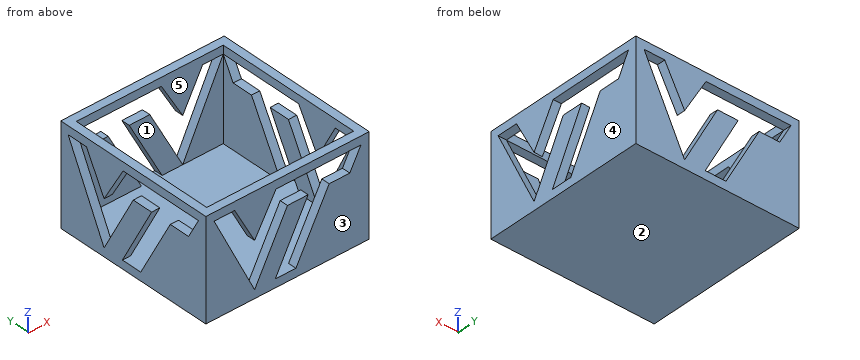
from build123d import *

# Parameters (mm, degrees)
F1_W      = 50.238024
F1_H      = 30.48
F2_DEPTH  = 50.2412
F4_T      = -2.54
F7_DEPTH  = 2.54
F8_DEPTH  = 2.54
F9_DEPTH  = 2.54
F10_DEPTH = 2.54


with BuildPart() as f2:
    # F1 (on Front) → F2 (new body)
    with BuildSketch(Plane.XZ):
        with Locations((7.288118, 12.7)):
            Rectangle(F1_W, F1_H)
    extrude(amount=-F2_DEPTH)

    # F4
    f4_openings = [f2.faces().sort_by_distance(p)[0] for p in [
        (7.288118, 25.1206, 27.94),
    ]]
    offset(amount=F4_T, openings=f4_openings)

    # F0 (on Front) → F7 (cut)
    with BuildSketch(Plane.XZ):
        Polygon((-8.940894, 25.4), (-15.290894, 25.4), (-2.829347, 0), (7.282625, 19.05), (13.632625, 19.05), (3.520653, 0), (9.870653, 0), (20.089414, 19.05), (26.439414, 19.05), (29.86713, 25.4), (3.759106, 25.4), (-2.829347, 13.97), align=None)
    extrude(amount=-F7_DEPTH, mode=Mode.SUBTRACT)

    # F6 (on face) → F8 (cut)
    with BuildSketch(Plane(origin=(-17.830894, 0, 0), x_dir=(0, -1, 0), z_dir=(-1, 0, 0))):
        Polygon((-41.3512, 25.4), (-47.7012, 25.4), (-35.239653, 0), (-25.127682, 19.05), (-18.777682, 19.05), (-28.889653, 0), (-22.539653, 0), (-12.320892, 19.05), (-5.970892, 19.05), (-2.543176, 25.4), (-28.6512, 25.4), (-35.239653, 13.97), align=None)
    extrude(amount=-F8_DEPTH, mode=Mode.SUBTRACT)

    # F5 (on face) → F9 (cut)
    with BuildSketch(Plane(origin=(0, 50.2412, 0), x_dir=(-1, 0, 0), z_dir=(0, 1, 0))):
        Polygon((-23.51713, 25.4), (-29.86713, 25.4), (-17.405583, 0), (-7.293612, 19.05), (-0.943612, 19.05), (-11.055583, 0), (-4.705583, 0), (5.513178, 19.05), (11.863178, 19.05), (15.290894, 25.4), (-10.81713, 25.4), (-17.405583, 13.97), align=None)
    extrude(amount=-F9_DEPTH, mode=Mode.SUBTRACT)

    # F3 (on face) → F10 (cut)
    with BuildSketch(Plane.YZ.offset(32.40713)):
        Polygon((8.89, 25.4), (2.54, 25.4), (15.001547, 0), (25.113518, 19.05), (31.463518, 19.05), (21.351547, 0), (27.701547, 0), (37.920308, 19.05), (44.270308, 19.05), (47.698024, 25.4), (21.59, 25.4), (15.001547, 13.97), align=None)
    extrude(amount=-F10_DEPTH, mode=Mode.SUBTRACT)


solid = f2.part
Model file for the job. Use its own axes, mm. Face numbers are marked on the shaded views. A direction names the side the tool comes from. Round coordinates to 2 decimals unless told otherwise and drop trailing zeros. Loops run counter-clockwise (first coordinate to the right, second up) from the corner with the lowest first, then second, coordinate; pieces in that order, holes last. Notation, with made-up numbers: M 15.25,76.5 L 51.25,76.5 A31 ccw 51.25,105.5 Z; hole C 16.25,75.25 d4. An arc over 180 degrees is marked long. One line per question, with ' | ' between items.
1) Drill centre lines: line 1 along Y through (x, z) = (-14.5, 1); line 2 along X through (y, z) = (13, 1); line 3 along Y through (x, z) = (30.5, 17). Where is each one in solid material? Low to high.
Solved:
line 1: y = 0 to 2.54, 47.7 to 50.24 | line 2: x = -17.83 to -15.29, 29.87 to 32.41 | line 3: y = 0 to 6.66, 13.38 to 16.75, 24.03 to 30.38, 36.82 to 50.24
2) Band-saw the part on A-A (x = -10.5). Give the cut face in (y, z).
Solved:
outline: M 0,-2.54 L 50.24,-2.54 L 50.24,19.05 L 47.7,19.05 L 47.7,0 L 2.54,0 L 2.54,15.63 L 0,15.63 Z; M 0,25.4 L 2.54,25.4 L 2.54,27.94 L 0,27.94 Z; M 47.7,25.4 L 50.24,25.4 L 50.24,27.94 L 47.7,27.94 Z
3) Band-saw the part on D-D (z = 4.5). Give the number of separate pieces and of enclosed holes in the cut face, then the cut area to 3 significant figures.
Solved:
separate pieces: 8 | enclosed holes: 0 | area: 373 mm²
4) Mould opens along X. For the marked faces 3, 4 and 5 say: +X half, -X half, draft (parallel to the pull), parting line (faces both ways), or undercut.
Solved:
face 3: draft | face 4: +X half | face 5: undercut
5) Band-saw the part on C-C (x = 12.5). Give the cut face in (y, z), then the cut area to 3 significant figures.
Solved:
outline: M 0,-2.54 L 50.24,-2.54 L 50.24,9.24 L 47.7,9.24 L 47.7,0 L 2.54,0 L 2.54,4.9 L 0,4.9 Z; M 0,16.92 L 2.54,16.92 L 2.54,19.05 L 0,19.05 Z; M 0,25.4 L 2.54,25.4 L 2.54,27.94 L 0,27.94 Z; M 47.7,22.48 L 50.24,22.48 L 50.24,27.94 L 47.7,27.94 Z | area: 189 mm²
6) 3-axis set-ups, long thin cutter, end or side, ignore diameter. For the marked faces 1 and 2: which of +Z, -Z, +X, -X, +Y, -Y reach the whole face in a straight line?
Solved:
face 1: +Z | face 2: -Z, +X, -X, +Y, -Y
7) Band-saw the part on B-B (y = 4.5). Give the cut face in (x, z) (3 decimals), then the cut area to 3 significant figures.
Solved:
outline: M -17.831,-2.54 L 32.407,-2.54 L 32.407,21.405 L 29.867,21.405 L 29.867,0 L -15.291,0 L -15.291,21.775 L -17.831,21.775 Z; M -17.831,25.4 L -15.291,25.4 L -15.291,27.94 L -17.831,27.94 Z; M 29.867,25.4 L 32.407,25.4 L 32.407,27.94 L 29.867,27.94 Z | area: 250 mm²
